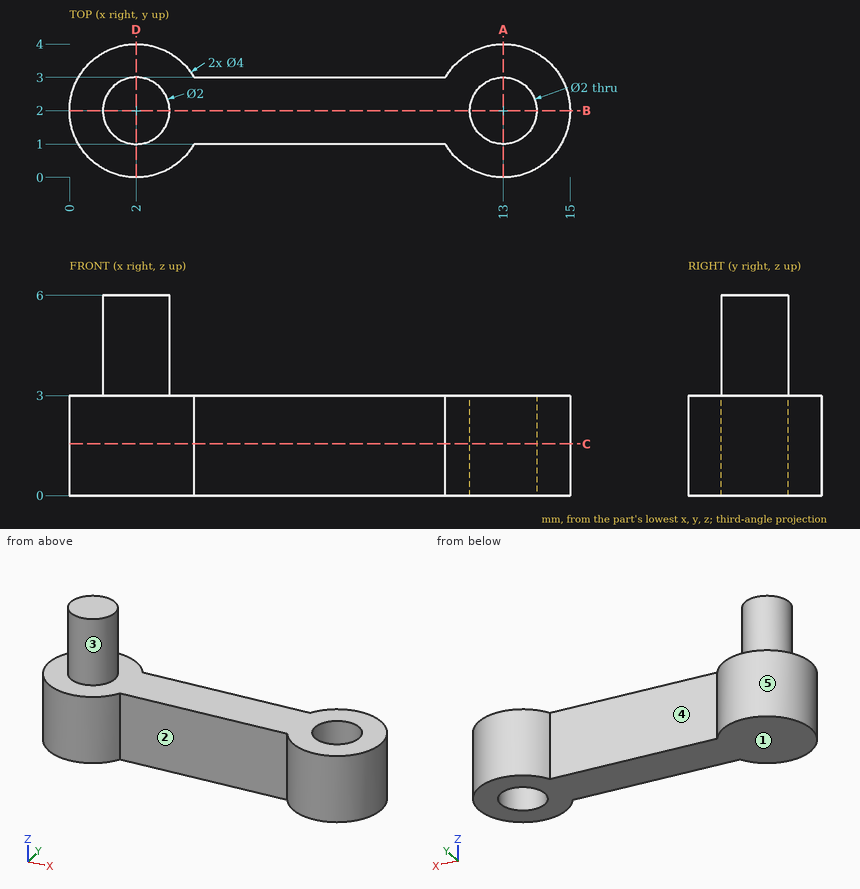
Design review of the part shown in the three views and the two pictorial views. Dimensions are in mm from the part's minimum x, y and z. A direction names the side the tool comes from. Give positions to 0.01 mm unless a question says otherwise; leave off trailing zeros. Order: outer loops, then holes, each group sorted by start corner. A loop starts at its lowest first (then second) coordinate and runs counter-clockwise, first axis right, second up. Notation, with made-up numbers: M 41,61 L 77,61 A15 ccw 77,69 Z; hole C 85.5,-26.5 d9. An arc over 180 degrees is marked long. Answer in a Markdown table with one row per item. Add a question column.
(1) Consider section B-B on y = 2. State the section outline as (x, z) points, and give its area (3 significant figures).
(2) For pin 1 (2 mm diameter, centred on y = 3.5, z = 1, fed in from -X); pin 2 (0.9 mm diameter, centred on x = 8, z = 1.5, fed in from -Y); pin 3 (0.9 mm diameter, centred on x = 6.5, z = 1, fed in from +Y); pin 4 (1.2 mm diameter, centred on x = 13, y = 2, fed in from -Z), all flat-tipped, find the tip position at first contact; note any pin that passes through.
(3) Wall thickness on probe 1 along Y at (x, z) = (13, 2.4); probe 2 along Z at (x, y) = (7.75, 1.3); probe 3 along Y at (x, z) = (4.75, 2.1): over which ranges is each line inside the solid? List them lowest first. Write a range as [from, to].
(4) Consider section C-C on z = 1.55. State the section outline as (x, y) points, and give its area (3 significant figures).
(5) Consider section D-D on x = 2. State the section outline as (y, z) points.
(6) Consider section A-A on x = 13. State the section outline as (y, z) points.
(7) For the marked faces 4 and 5, list the 3-axis set-ups (+Z, -Z, +X, -X, +Y, -Y) from which the entire face can be reached by the end or side of a thin tool; tool diameter is ignored.
(8) Mouldability with a two-part tool opening along X and no side actions: class the marked faces 1, 2 and 3 as +X half, -X half, draft (parallel to the pull), parting line (faces both ways), or undercut.
Evaluation:
| question | item | result |
|---|---|---|
| 1 | outline | M 0,0 L 12,0 L 12,3 L 3,3 L 3,6 L 1,6 L 1,3 L 0,3 Z; M 14,0 L 15,0 L 15,3 L 14,3 Z |
| 1 | area | 45.0 mm^2 |
| 2 | pin 1 | stops at x = 0.06 |
| 2 | pin 2 | stops at y = 1 |
| 2 | pin 3 | stops at y = 3 |
| 2 | pin 4 | passes through |
| 3 | probe 1 | y = [0, 1], [3, 4] |
| 3 | probe 2 | z = [0, 3] |
| 3 | probe 3 | y = [1, 3] |
| 4 | outline | M 3.73,1 L 11.27,1 A2 ccw long 11.27,3 L 3.73,3 A2 ccw long Z; hole C 13,2 d2 |
| 4 | area | 36.3 mm^2 |
| 5 | outline | M 0,0 L 4,0 L 4,3 L 3,3 L 3,6 L 1,6 L 1,3 L 0,3 Z |
| 6 | outline | M 0,0 L 1,0 L 1,3 L 0,3 Z; M 3,0 L 4,0 L 4,3 L 3,3 Z |
| 7 | face 4 | +Z, -Z, +Y |
| 7 | face 5 | +Z, -Z |
| 8 | face 1 | draft |
| 8 | face 2 | undercut |
| 8 | face 3 | parting line |
